The model under review builds one solid part; all positions refer to its coordinate system, in mm. Face numbers are marked on the shaded views. A direction names the side the tool comes from. Round coordinates to 2 decimals unless told otherwise and drop trailing zeros. Order: outer loops, then holes, each group sorted by start corner. A loop starts at its lowest first (then second) coordinate and runs counter-clockwise, first axis right, second up. Notation, with made-up numbers: M 25,38 L 41,38 A15 cw 41,65 Z; hole C -27.75,52.25 d7. An arc over 180 degrees is marked long. Answer as a JSON object with one key per item and string values. Group by question number.
1. Add section D-D on x = -45.5. Give the number of separate pieces and of enclosed holes in the cut face, and give its area (3 significant figures).
2. Add section C-C on x = 1. State the section outline as (y, z) points, and give its area (3 significant figures).
3. Clearance check with flat-ended pins moving along their axes: P1, Ø8, axis at x = -48, y = 26.5, coming from the +Z side; P2, Ø5, axis at x = -50.5, y = 30, coming from the -Z side; P3, Ø12, axis at x = -35, z = -9.5, coming from the +Y side. State where each tip first meets the part, or that it passes through.
4. Add section B-B on z = 57.15. State the section outline as (x, y) points.
5. Add section A-A on y = 12. State the section outline as (x, z) points.
6. Mouldability with a two-part tool opening along X and no side actions: class the marked faces 3, 4 and 5 as released by +X, released by -X, zero draft, split by the parting line, or undercut.
7. Machinability: for the marked faces 1 and 2, which of the approach directions +Z, -Z, +X, -X, +Y, -Y give a long, thin tool a straight path to every point of the face, cutting with its end or side? Answer none if there is none.
8. To check wall thickness, follow probe 1 along Y at (x, z) = (-49, 0); probe 2 along Y at (x, z) = (-16, -12.5); probe 3 along X at (y, z) = (6, -7). State the ranges of each line that lie inside material, in increasing order. Write a range as [from, to].
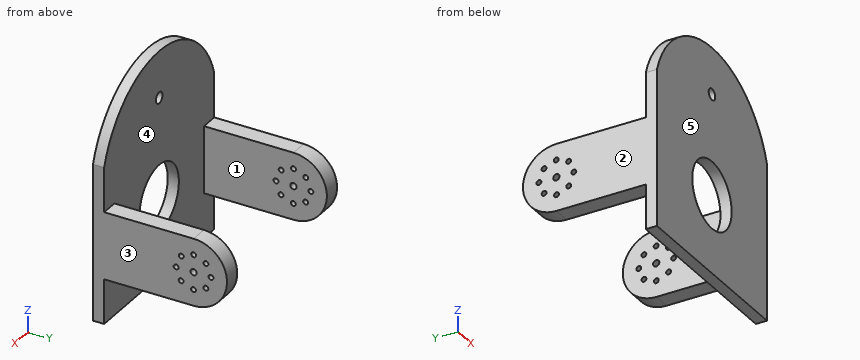
```python
from build123d import *

# Parameters (mm, degrees)
SKETCH1_R           = 19.05
SKETCH1_R_2         = 3.175
BOSS_EXTRUDE1_DEPTH = 6.35
SKETCH6_W           = 9.906
SKETCH6_H           = 38.1
BOSS_EXTRUDE2_DEPTH = 76.2
SKETCH7_R           = 1.397
SKETCH7_R_2         = 1.7859375
CUT_EXTRUDE1_DEPTH  = 107.68


with BuildPart() as part:
    # Sketch1 → Boss-Extrude1 (new body)
    with BuildSketch(Plane(origin=(0, 0, 0), x_dir=(1, 0, 0), z_dir=(0, 1, 0))):
        with BuildLine():
            Line((-53.503176773, 44.45), (53.176823227, 44.45))
            Line((53.176823227, 44.45), (53.176823227, -44.45))
            ThreePointArc((53.176823227, -44.45), (-0.163176773, -83.674106148), (-53.503176773, -44.45))
            Line((-53.503176773, -44.45), (-53.503176773, 44.45))
        make_face()
        with Locations((-0.163176773, 0)):
            Circle(SKETCH1_R, mode=Mode.SUBTRACT)
        with Locations((-0.163176773, -57.15)):
            Circle(SKETCH1_R_2, mode=Mode.SUBTRACT)
    extrude(amount=BOSS_EXTRUDE1_DEPTH)

    # Sketch6 → Boss-Extrude2 (add)
    with BuildSketch(Plane(origin=(0, 6.35, 0), x_dir=(1, 0, 0), z_dir=(0, 1, 0))):
        with Locations((-48.550176773, 0)):
            Rectangle(SKETCH6_W, SKETCH6_H)
        with Locations((48.223823227, 0)):
            Rectangle(SKETCH6_W, SKETCH6_H)
    extrude(amount=BOSS_EXTRUDE2_DEPTH)

    # Sketch7 → Cut-Extrude1 (cut, through all)
    with BuildSketch(Plane.ZY.offset(53.503176773)):
        with Locations((-6.991480211, 64.122926346)):
            Circle(SKETCH7_R)
        with Locations((0, 67.056)):
            Circle(SKETCH7_R)
        with Locations((7.017719338, 64.186273203)):
            Circle(SKETCH7_R)
        with Locations((9.950792993, 57.194792993)):
            Circle(SKETCH7_R)
        with Locations((7.081066196, 50.177073654)):
            Circle(SKETCH7_R)
        with Locations((0.089585985, 47.244)):
            Circle(SKETCH7_R)
        with Locations((-6.928133353, 50.113726797)):
            Circle(SKETCH7_R)
        with Locations((-9.861207007, 57.105207007)):
            Circle(SKETCH7_R)
        with Locations((0.044792993, 57.15)):
            Circle(SKETCH7_R_2)
        with BuildLine():
            Line((-19.05, 57.105207007), (-19.05, 82.55))
            Line((-19.05, 82.55), (19.05, 82.55))
            Line((19.05, 82.55), (19.05, 57.194792993))
            ThreePointArc((19.05, 57.194792993), (-0.044687793, 76.155259669), (-19.05, 57.105207007))
        make_face()
    extrude(amount=-CUT_EXTRUDE1_DEPTH, mode=Mode.SUBTRACT)


solid = part.part
```
Recorded:
{
 "1": {"separate pieces": "1", "enclosed holes": "9", "area": "3,110 mm²"},
 "2": {"outline": "M 0,-44.45 L 6.35,-44.45 L 6.35,-19.01 L 0,-19.01 Z; M 0,19.01 L 6.35,19.01 L 6.35,54.2 L 0,54.2 Z; M 0,60.1 L 6.35,60.1 L 6.35,83.66 L 0,83.66 Z", "area": "535 mm²"},
 "3": {"P1": "stops at z = 19.05", "P2": "stops at z = -19.05", "P3": "stops at y = 6.35"},
 "4": {"outline": "M -47.71,0 L -3.34,0 L -3.34,6.35 L -47.71,6.35 Z; M 3.01,0 L 47.38,0 L 47.38,6.35 L 3.01,6.35 Z"},
 "5": {"outline": "M -53.5,-19.05 L -43.6,-19.05 L -43.6,19.05 L -53.5,19.05 Z; M 43.27,-19.05 L 53.18,-19.05 L 53.18,19.05 L 43.27,19.05 Z"},
 "6": {"face 3": "released by +X", "face 4": "undercut", "face 5": "zero draft"},
 "7": {"face 1": "+Z, -Z, +Y", "face 2": "+Z, -Z, -X, +Y, -Y"},
 "8": {"probe 1": "y = [0, 45.85], [48.64, 55.36], [58.94, 65.66], [68.45, 76.16]", "probe 2": "y = [0, 6.35]", "probe 3": "x = [-53.5, -17.88], [17.55, 53.18]"}
}
